Source: CAD feature listing. Evaluate the final solid. Frame: model axes, mm. A direction names the side the tool comes from. Coordinates: 2 decimals unless noted, no trailing zeros. Write each loop counter-clockwise with the first axis right and the second up, starting at its lowest first coordinate (ties: lowest second). Pieces come first, ordered by that corner, then holes. Notation, with made-up numbers: (0.25, 68.25) - (28.25, 68.25) arc R23 cw to (28.25, 79.25) - close; hole circle Ø8 at (48, 20). An arc over 180 degrees is marked (long way). One line per question, with ' | ' between items. Start each with the question number.
Q1. Draft query along Z for faces 3 (the face through (-4.7, 38.268, 8.3)), 4 (the face through (-8, 5.66, 2.11)), 5 (the face through (6.75, 18.94, -10.58)). Return one class per face: +Z half, -Z half, draft (parallel to the pull), parting line (faces both ways), or undercut.
Q2. Line query: line 1 (X direction, y = 16, z = 0); line 2 (Z direction, x = 0, y = 53.25) (3 decimals). Output: solid intervals per line, ascending.
Q3. Contact query for flat-ended pins moving along their axis: P1, Ø4, axis at x = 7, y = 17.5, coming from the -Z side; P2, Ø0.7, axis at y = 5.5, z = -3.5, coming from the +X side; P3, Ø4, axis at y = 38.5, z = -8.5, coming from the +X side. Output: stop coordinate, or through.
Q4. Access query for faces 1 (the face through (-7.15, 6, -4)), 2 (the face through (0, 49.698, 0)). Directions: +Z, -Z, +X, -X, +Y, -Y. A direction counts if a zero-diameter tool reaches every point of the face in a straight line with its end or side. Return the directions, or none.
Q5. Cut plane D-D, the plane z = -4. Return loops of the section in (x, y).
Q6. Cut plane C-C, the plane y = 25.5. Return loops of the section in (x, z).
```python
from build123d import *

# Parameters (mm, degrees)
SKETCH1_R            = 12.7
BOSS_EXTRUDE1_DEPTH  = 38.4175
SKETCH4_R            = 9.525
BOSS_EXTRUDE2_DEPTH  = 17.78
CUT_EXTRUDE1_DEPTH   = 11.176
SKETCH3_R            = 6
CUT_EXTRUDE2_DEPTH   = 8
SKETCH6_R            = 3.1496
CUT_EXTRUDE3_DEPTH   = 6.35
SPLIT1_START         = 11.325999954
SPLIT1_OUTLINE_R     = 12.550000046
SPLIT1_OUTLINE_R_2   = 6.149999954
SPLIT1_DEPTH         = 26.941500092
SPLIT1_START_2       = 19.325999954
SPLIT1_2_OUTLINE_R   = 9.375000046
SPLIT1_2_OUTLINE_R_2 = 3.299599954
SPLIT1_2_DEPTH       = 36.721500092
SPLIT1_START_3       = 0.149999954
SPLIT1_3_OUTLINE_R   = 12.550000046
SPLIT1_3_DEPTH       = 11.176
SPLIT1_4_OUTLINE_R   = 3.299599954
SPLIT1_4_DEPTH       = 30.371500092
SPLIT1_5_OUTLINE_R   = 12.550000046
SPLIT1_5_OUTLINE_R_2 = 6.149999954
SPLIT1_5_DEPTH       = 26.941500092
SPLIT1_6_OUTLINE_R   = 9.375000046
SPLIT1_6_OUTLINE_R_2 = 3.299599954
SPLIT1_6_DEPTH       = 36.721500092
SPLIT1_7_OUTLINE_R   = 12.550000046
SPLIT1_7_DEPTH       = 11.176
SPLIT1_8_OUTLINE_R   = 3.299599954
SPLIT1_8_DEPTH       = 30.371500092


with BuildPart() as part:
    # Sketch1 → Boss-Extrude1 (new body)
    with BuildSketch(Plane(origin=(0, 0, 0), x_dir=(1, 0, 0), z_dir=(0, 1, 0))):
        with Locations(Location((0, 0, 0), (0, 0, 270))):
            Circle(SKETCH1_R)
    extrude(amount=BOSS_EXTRUDE1_DEPTH)

    # Sketch4 → Boss-Extrude2 (add)
    with BuildSketch(Plane(origin=(0, 38.4175, 0), x_dir=(1, 0, 0), z_dir=(0, 1, 0))):
        with Locations(Location((0, 0, 0), (0, 0, 270))):
            Circle(SKETCH4_R)
    extrude(amount=BOSS_EXTRUDE2_DEPTH)

    # Sketch2 → Cut-Extrude1 (cut)
    with BuildSketch(Plane.XZ):
        with BuildLine():
            Line((-7, 2.899494937), (-8.776962921, 1.122532015))
            ThreePointArc((-8.776962921, 1.122532015), (-9.241930906, 0), (-8.776962921, -1.122532015))
            Line((-8.776962921, -1.122532015), (-7, -2.899494937))
            Line((-7, -2.899494937), (-7, 2.899494937))
        make_face()
        Polygon((-2.899494937, 7), (-7, 2.899494937), (-7, -2.899494937), (-2.899494937, -7), (2.899494937, -7), (7, -2.899494937), (7, 2.899494937), (2.899494937, 7), align=None)
        with BuildLine():
            Line((-7, 5.4125), (-7, 2.899494937))
            Line((-7, 2.899494937), (-2.899494937, 7))
            Line((-2.899494937, 7), (-5.4125, 7))
            ThreePointArc((-5.4125, 7), (-6.535032015, 6.535032015), (-7, 5.4125))
        make_face()
        with BuildLine():
            Line((-1.122532015, 8.776962921), (-2.899494937, 7))
            Line((-2.899494937, 7), (2.899494937, 7))
            Line((2.899494937, 7), (1.122532015, 8.776962921))
            ThreePointArc((1.122532015, 8.776962921), (0, 9.241930906), (-1.122532015, 8.776962921))
        make_face()
        with BuildLine():
            Line((5.4125, 7), (2.899494937, 7))
            Line((2.899494937, 7), (7, 2.899494937))
            Line((7, 2.899494937), (7, 5.4125))
            ThreePointArc((7, 5.4125), (6.535032015, 6.535032015), (5.4125, 7))
        make_face()
        with BuildLine():
            Line((8.776962921, 1.122532015), (7, 2.899494937))
            Line((7, 2.899494937), (7, -2.899494937))
            Line((7, -2.899494937), (8.776962921, -1.122532015))
            ThreePointArc((8.776962921, -1.122532015), (9.241930906, 0), (8.776962921, 1.122532015))
        make_face()
        with BuildLine():
            Line((7, -2.899494937), (2.899494937, -7))
            Line((2.899494937, -7), (5.4125, -7))
            ThreePointArc((5.4125, -7), (6.535032015, -6.535032015), (7, -5.4125))
            Line((7, -5.4125), (7, -2.899494937))
        make_face()
        with BuildLine():
            Line((2.899494937, -7), (-2.899494937, -7))
            Line((-2.899494937, -7), (-1.122532015, -8.776962921))
            ThreePointArc((-1.122532015, -8.776962921), (0, -9.241930906), (1.122532015, -8.776962921))
            Line((1.122532015, -8.776962921), (2.899494937, -7))
        make_face()
        with BuildLine():
            Line((-2.899494937, -7), (-7, -2.899494937))
            Line((-7, -2.899494937), (-7, -5.4125))
            ThreePointArc((-7, -5.4125), (-6.535032015, -6.535032015), (-5.4125, -7))
            Line((-5.4125, -7), (-2.899494937, -7))
        make_face()
    extrude(amount=-CUT_EXTRUDE1_DEPTH, mode=Mode.SUBTRACT)

    # Sketch3 → Cut-Extrude2 (cut)
    with BuildSketch(Plane.XZ.offset(-11.176)):
        with Locations(Location((0, 0, 0), (0, 0, 270))):
            Circle(SKETCH3_R)
    extrude(amount=-CUT_EXTRUDE2_DEPTH, mode=Mode.SUBTRACT)

    # Sketch6 → Cut-Extrude3 (cut)
    with BuildSketch(Plane(origin=(0, 56.1975, 0), x_dir=(1, 0, 0), z_dir=(0, 1, 0))):
        with Locations(Location((0, 0, 0), (0, 0, 270))):
            Circle(SKETCH6_R)
    extrude(amount=-CUT_EXTRUDE3_DEPTH, mode=Mode.SUBTRACT)

    # Split1 5 outline → Split1 5 (cut)
    with BuildSketch(Plane(origin=(0, 0, 0), x_dir=(1, 0, 0), z_dir=(0, 1, 0)).offset(SPLIT1_START)):
        Circle(SPLIT1_5_OUTLINE_R)
        Circle(SPLIT1_5_OUTLINE_R_2, mode=Mode.SUBTRACT)
    extrude(amount=SPLIT1_5_DEPTH, mode=Mode.SUBTRACT)

    # Split1 6 outline → Split1 6 (cut)
    with BuildSketch(Plane(origin=(0, 0, 0), x_dir=(1, 0, 0), z_dir=(0, 1, 0)).offset(SPLIT1_START_2)):
        Circle(SPLIT1_6_OUTLINE_R)
        Circle(SPLIT1_6_OUTLINE_R_2, mode=Mode.SUBTRACT)
    extrude(amount=SPLIT1_6_DEPTH, mode=Mode.SUBTRACT)

    # Split1 7 outline → Split1 7 (cut)
    with BuildSketch(Plane(origin=(0, 0, 0), x_dir=(1, 0, 0), z_dir=(0, 1, 0)).offset(SPLIT1_START_3)):
        Circle(SPLIT1_7_OUTLINE_R)
        with BuildLine():
            Line((-7.149999954, -2.961626952), (-8.883028906, -1.228598))
            ThreePointArc((-8.883028906, -1.228598), (-9.39193086, 0), (-8.883028906, 1.228598))
            Line((-8.883028906, 1.228598), (-7.149999954, 2.961626952))
            Line((-7.149999954, 2.961626952), (-7.149999954, 5.4125))
            ThreePointArc((-7.149999954, 5.4125), (-6.641098, 6.641098), (-5.4125, 7.149999954))
            Line((-5.4125, 7.149999954), (-2.961626952, 7.149999954))
            Line((-2.961626952, 7.149999954), (-1.228598, 8.883028906))
            ThreePointArc((-1.228598, 8.883028906), (0, 9.39193086), (1.228598, 8.883028906))
            Line((1.228598, 8.883028906), (2.961626952, 7.149999954))
            Line((2.961626952, 7.149999954), (5.4125, 7.149999954))
            ThreePointArc((5.4125, 7.149999954), (6.641098, 6.641098), (7.149999954, 5.4125))
            Line((7.149999954, 5.4125), (7.149999954, 2.961626952))
            Line((7.149999954, 2.961626952), (8.883028906, 1.228598))
            ThreePointArc((8.883028906, 1.228598), (9.39193086, 0), (8.883028906, -1.228598))
            Line((8.883028906, -1.228598), (7.149999954, -2.961626952))
            Line((7.149999954, -2.961626952), (7.149999954, -5.4125))
            ThreePointArc((7.149999954, -5.4125), (6.641098, -6.641098), (5.4125, -7.149999954))
            Line((5.4125, -7.149999954), (2.961626952, -7.149999954))
            Line((2.961626952, -7.149999954), (1.228598, -8.883028906))
            ThreePointArc((1.228598, -8.883028906), (0, -9.39193086), (-1.228598, -8.883028906))
            Line((-1.228598, -8.883028906), (-2.961626952, -7.149999954))
            Line((-2.961626952, -7.149999954), (-5.4125, -7.149999954))
            ThreePointArc((-5.4125, -7.149999954), (-6.641098, -6.641098), (-7.149999954, -5.4125))
            Line((-7.149999954, -5.4125), (-7.149999954, -2.961626952))
        make_face(mode=Mode.SUBTRACT)
    extrude(amount=SPLIT1_7_DEPTH, mode=Mode.SUBTRACT)

    # Split1 8 outline → Split1 8 (cut)
    with BuildSketch(Plane(origin=(0, 0, 0), x_dir=(1, 0, 0), z_dir=(0, 1, 0)).offset(SPLIT1_START_2)):
        Circle(SPLIT1_8_OUTLINE_R)
    extrude(amount=SPLIT1_8_DEPTH, mode=Mode.SUBTRACT)


with BuildPart() as body_2:
    # Split1: read off the stored shape, not the designer's step
    # Split1 outline → Split1 (new body)
    with BuildSketch(Plane(origin=(0, 0, 0), x_dir=(1, 0, 0), z_dir=(0, 1, 0)).offset(SPLIT1_START)):
        Circle(SPLIT1_OUTLINE_R)
        Circle(SPLIT1_OUTLINE_R_2, mode=Mode.SUBTRACT)
    extrude(amount=SPLIT1_DEPTH)

    # Split1 2 outline → Split1 2 (add)
    with BuildSketch(Plane(origin=(0, 0, 0), x_dir=(1, 0, 0), z_dir=(0, 1, 0)).offset(SPLIT1_START_2)):
        Circle(SPLIT1_2_OUTLINE_R)
        Circle(SPLIT1_2_OUTLINE_R_2, mode=Mode.SUBTRACT)
    extrude(amount=SPLIT1_2_DEPTH)

    # Split1 3 outline → Split1 3 (add)
    with BuildSketch(Plane(origin=(0, 0, 0), x_dir=(1, 0, 0), z_dir=(0, 1, 0)).offset(SPLIT1_START_3)):
        Circle(SPLIT1_3_OUTLINE_R)
        with BuildLine():
            Line((7.149999954, 5.4125), (7.149999954, 2.961626952))
            Line((7.149999954, 2.961626952), (8.883028906, 1.228598))
            ThreePointArc((8.883028906, 1.228598), (9.39193086, 0), (8.883028906, -1.228598))
            Line((8.883028906, -1.228598), (7.149999954, -2.961626952))
            Line((7.149999954, -2.961626952), (7.149999954, -5.4125))
            ThreePointArc((7.149999954, -5.4125), (6.641098, -6.641098), (5.4125, -7.149999954))
            Line((5.4125, -7.149999954), (2.961626952, -7.149999954))
            Line((2.961626952, -7.149999954), (1.228598, -8.883028906))
            ThreePointArc((1.228598, -8.883028906), (0, -9.39193086), (-1.228598, -8.883028906))
            Line((-1.228598, -8.883028906), (-2.961626952, -7.149999954))
            Line((-2.961626952, -7.149999954), (-5.4125, -7.149999954))
            ThreePointArc((-5.4125, -7.149999954), (-6.641098, -6.641098), (-7.149999954, -5.4125))
            Line((-7.149999954, -5.4125), (-7.149999954, -2.961626952))
            Line((-7.149999954, -2.961626952), (-8.883028906, -1.228598))
            ThreePointArc((-8.883028906, -1.228598), (-9.39193086, 0), (-8.883028906, 1.228598))
            Line((-8.883028906, 1.228598), (-7.149999954, 2.961626952))
            Line((-7.149999954, 2.961626952), (-7.149999954, 5.4125))
            ThreePointArc((-7.149999954, 5.4125), (-6.641098, 6.641098), (-5.4125, 7.149999954))
            Line((-5.4125, 7.149999954), (-2.961626952, 7.149999954))
            Line((-2.961626952, 7.149999954), (-1.228598, 8.883028906))
            ThreePointArc((-1.228598, 8.883028906), (0, 9.39193086), (1.228598, 8.883028906))
            Line((1.228598, 8.883028906), (2.961626952, 7.149999954))
            Line((2.961626952, 7.149999954), (5.4125, 7.149999954))
            ThreePointArc((5.4125, 7.149999954), (6.641098, 6.641098), (7.149999954, 5.4125))
        make_face(mode=Mode.SUBTRACT)
    extrude(amount=SPLIT1_3_DEPTH)

    # Split1 4 outline → Split1 4 (add)
    with BuildSketch(Plane(origin=(0, 0, 0), x_dir=(1, 0, 0), z_dir=(0, 1, 0)).offset(SPLIT1_START_2)):
        Circle(SPLIT1_4_OUTLINE_R)
    extrude(amount=SPLIT1_4_DEPTH)


solid = body_2.part
```
Reply:
1) face 3: draft | face 4: undercut | face 5: parting line
2) line 1: x = -12.55 to -6.15, 6.15 to 12.55 | line 2: z = -9.375 to -3.3, 3.3 to 9.375
3) P1: stops at z = -11.51 | P2: stops at x = 12.15 | P3: stops at x = 10.73
4) face 1: -Y | face 2: +Y
5) outline: (-11.9, 0.15) - (-7.15, 0.15) - (-7.15, 11.33) - (-4.67, 11.33) - (-4.67, 19.33) - (4.67, 19.33) - (4.67, 11.33) - (7.15, 11.33) - (7.15, 0.15) - (11.9, 0.15) - (11.9, 38.27) - (8.48, 38.27) - (8.48, 56.05) - (-8.48, 56.05) - (-8.48, 38.27) - (-11.9, 38.27) - close
6) outline: circle Ø25.1 at (0, 0)
